Read the model definition and answer for the solid it produces. Units are mm, in the model's axes. A direction names the side the tool comes from. Give positions to 0.01 mm unless a question says otherwise; leave off trailing zeros. Order: outer loops, then holes, each group sorted by start corner. A loop starts at its lowest first (then second) coordinate and runs counter-clockwise, first axis right, second up. Notation, with made-up numbers: (-36.75, -17) - (3.25, -17) arc R8 cw to (3.25, -7) - close; hole circle Ø4 at (-33.75, 23). An arc over 180 degrees is marked (long way). Write each question's results on one line, items separated by ' | '.
from build123d import *

# Parameters (mm, degrees)
F0_R     = 2.5
F1_DEPTH = 50
F2_R     = 4.2
F3_DEPTH = 5
F4_R     = 5
F5_DEPTH = 1


with BuildPart() as f1:
    # F0 (on Top) → F1 (new body)
    with BuildSketch(Plane.XY):
        Circle(F0_R)
    extrude(amount=-F1_DEPTH)

    # F2 (on Top) → F3 (join)
    with BuildSketch(Plane.XY):
        Circle(F2_R)
    extrude(amount=F3_DEPTH)

    # F4 (on Top) → F5 (join)
    with BuildSketch(Plane.XY):
        Circle(F4_R)
    extrude(amount=-F5_DEPTH)


solid = f1.part
(1) Section A-A (y = 0) is taken. Give the vertices of the cut face in (x, z), plus the area to 3 significant figures.
Conclusion:
outline: (-5, -1) - (-2.5, -1) - (-2.5, -50) - (2.5, -50) - (2.5, -1) - (5, -1) - (5, 0) - (4.2, 0) - (4.2, 5) - (-4.2, 5) - (-4.2, 0) - (-5, 0) - close | area: 297 mm^2
(2) Section D-D (y = -3.5) is taken. Give the vertices of the cut face in (x, z), plus the area to 3 significant figures.
Conclusion:
outline: (-3.57, -1) - (3.57, -1) - (3.57, 0) - (2.32, 0) - (2.32, 5) - (-2.32, 5) - (-2.32, 0) - (-3.57, 0) - close | area: 30.4 mm^2
(3) Section C-C (z = -3) is taken. Give the vertices of the cut face in (x, y).
Conclusion:
outline: circle Ø5 at (0, 0)
(4) Consider probe 1 along Z at (x, y) = (-3.5, -2.5); probe 2 along Z at (x, y) = (-1, 3); probe 3 along Y at (x, z) = (-2, -5.5). Determine where each line is inside the solid, lowest interval first. Write a range as [from, to].
Conclusion:
probe 1: [-1, 0] | probe 2: [-1, 5] | probe 3: [-1.5, 1.5]
(5) For faces 1 (the face through (0, 0, -50)), 2 (the face through (4.006, 1.262, 2.465)), 3 (the face through (-0.54, -2.44, -25.16)), determine the directions among +Z, -Z, +X, -X, +Y, -Y from which every point of the face is accessible in a straight line to the end or side of a thin tool.
Conclusion:
face 1: -Z, +X, -X, +Y, -Y | face 2: +Z | face 3: -Z
(6) Each of these flat-tipped pins is pushed along its axis until it touches: pin 1 (2 mm diameter, centred on x = 0.5, z = -28.5, fed in from -Y); pin 2 (6 mm diameter, centred on y = -2, z = -25.5, fed in from -X); pin 3 (6 mm diameter, centred on x = -4, z = -6, fed in from -Y). Where does it stop, or does it pass through?
Conclusion:
pin 1: y = -2.5 | pin 2: x = -2.5 | pin 3: y = -2.29
